Source: three-view drawing plus pictorial views. Frame: mm from the lowest corner of the part. A direction names the side the tool comes from. Round coordinates to 2 decimals unless told otherwise and drop trailing zeros. Order: outer loops, then holes, each group sorted by start corner. A loop starts at its lowest first (then second) coordinate and runs counter-clockwise, first axis right, second up. Notation, with made-up numbers: (-12.5, -37) -> (23.5, -37) arc R30 ccw to (23.5, -9) -> close; hole circle Ø4 at (-0.5, 21.25). An arc over 180 degrees is marked (long way). Answer as CSV lines item,"result". Start each with the question number.
1) Mould query, pull axis X, two halves, no side actions, for the marked faces 4, 5 and 6. Classes: +X half, -X half, draft (parallel to the pull), parting line (faces both ways), or undercut.
2) Section query C-C, the plane x = 16. Output: boundary loops of the cut face in (y, z).
3) Section query A-A, the plane y = 12. Output: boundary loops of the cut face in (x, z), and give its area (3 significant figures).
4) Access query for the marked faces 1, 2 and 3. Directions: +Z, -Z, +X, -X, +Y, -Y. A direction counts if a zero-diameter tool reaches every point of the face in a straight line with its end or side. Return the directions, or none.
5) First-contact query: P1, Ø1, axis at y = 12, z = 10, coming from the -X side; P2, Ø8, axis at x = 36.5, z = 12.5, coming from the -Y side; P3, Ø6, axis at y = 24, z = 17.5, coming from the -X side. Flat tips, straight axial feed; report the tip coordinate or a pass-through.
6) Line query: L1, parallel to Z at x = 16, y = 34; L2, parallel to X at y = 13, z = 1; L3, parallel to Y at x = 26.5, z = 4. Output: solid intervals per line, ascending.
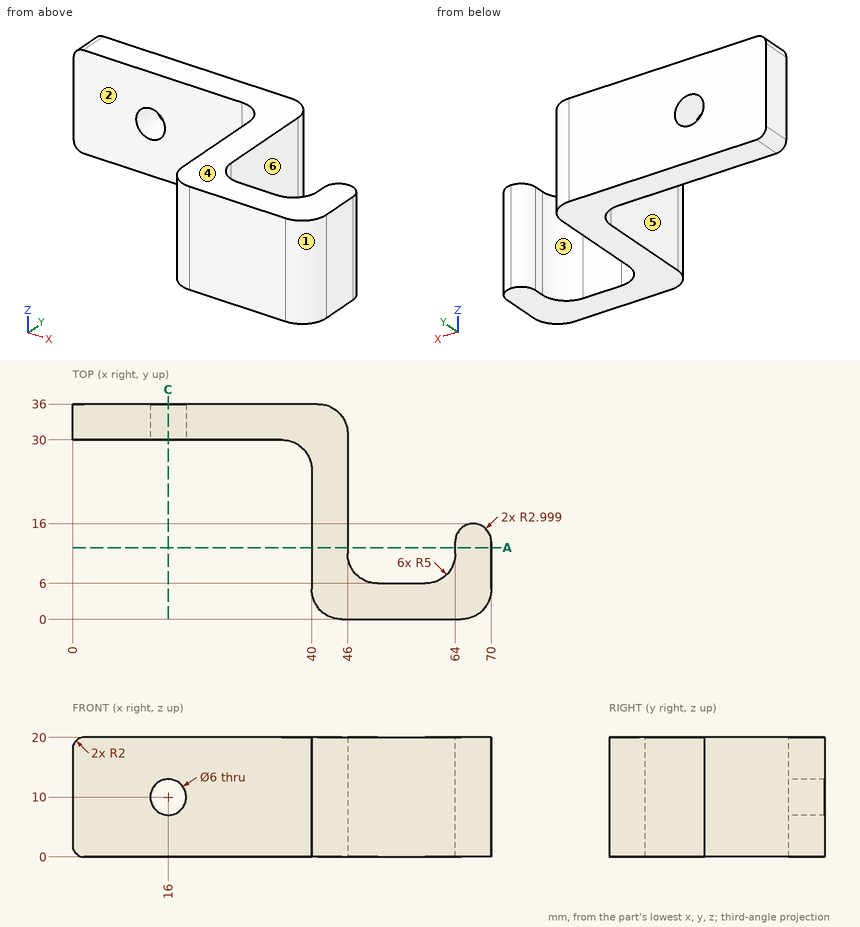
Findings:
1,face 4,"draft"
1,face 5,"-X half"
1,face 6,"undercut"
2,outline,"(30, 0) -> (36, 0) -> (36, 7) -> (30, 7) -> close; (30, 13) -> (36, 13) -> (36, 20) -> (30, 20) -> close"
3,outline,"(40, 0) -> (46, 0) -> (46, 20) -> (40, 20) -> close; (64, 0) -> (70, 0) -> (70, 20) -> (64, 20) -> close"
3,area,"240 mm^2"
4,face 1,"+Z, -Z, +X, -Y"
4,face 2,"+Z, -Z, -X, -Y"
4,face 3,"+Z, -Z, +Y"
5,P1,"stops at x = 40"
5,P2,"stops at y = 2.82"
5,P3,"stops at x = 39.58"
6,L1,"z = 0 to 7, 13 to 20"
6,L2,"x = 40 to 46, 64 to 70"
6,L3,"y = 30 to 36"
